from build123d import *

# Parameters (mm, degrees)
SKETCH_1_W             = 580
SKETCH_1_H             = 285
EXTRUDE_1_DEPTH        = 10
HOLE_WIZARD_M5_1_D     = 4.2
HOLE_WIZARD_M5_2_D     = 4.2
HOLE_WIZARD_M5_3_D     = 4.2
SKETCH_11_W            = 330
SKETCH_11_H            = 80
CUT_EXTRUDE_1_DEPTH    = 2
HOLE_WIZARD_M5_4_D     = 4.2
HOLE_WIZARD_M5_4_DEPTH = 2
HOLE_WIZARD_M5_4_TIP   = 1.2618073


with BuildPart() as part:
    # 草图1 → 凸台-拉伸1 (new body)
    with BuildSketch(Plane.XY):
        Rectangle(SKETCH_1_W, SKETCH_1_H)
    extrude(amount=EXTRUDE_1_DEPTH)

    # M5 螺纹孔1 (through all)
    with Locations(Plane(origin=(290, 0, 0), x_dir=(0, 0, -1), z_dir=(1, 0, 0))):
        with Locations((-5, 125), (-5, 75), (-5, 25), (-5, -25), (-5, -75), (-5, -125)):
            Hole(HOLE_WIZARD_M5_1_D / 2)

    # M5 螺纹孔2 (through all)
    with Locations(Plane(origin=(0, 142.5, 0), x_dir=(1, 0, 0), z_dir=(0, 1, 0))):
        with Locations((0, -5), (50, -5)):
            Hole(HOLE_WIZARD_M5_2_D / 2)

    # M5 螺纹孔3 (through all)
    with Locations(Plane.XY.offset(10)):
        with Locations((-160, -132.5), (-80, -132.5), (80, -132.5), (160, -132.5)):
            Hole(HOLE_WIZARD_M5_3_D / 2)

    # 草图11 → 切除-拉伸1 (cut)
    with BuildSketch(Plane(origin=(0, 0, 0), x_dir=(-1, 0, 0), z_dir=(0, 0, -1))):
        with Locations((0, 87.5)):
            Rectangle(SKETCH_11_W, SKETCH_11_H)
    extrude(amount=-CUT_EXTRUDE_1_DEPTH, mode=Mode.SUBTRACT)

    # M5 螺纹孔4
    with Locations(Plane(origin=(0, 0, 2), x_dir=(-1, 0, 0), z_dir=(0, 0, -1))):
        with Locations((-155, 119.5), (-155, 55.5), (155, 55.5), (155, 119.5)):
            Hole(HOLE_WIZARD_M5_4_D / 2, depth=HOLE_WIZARD_M5_4_DEPTH)
            with Locations((0, 0, -(HOLE_WIZARD_M5_4_DEPTH + HOLE_WIZARD_M5_4_TIP / 2))):  # 118° drill point
                Cone(0, HOLE_WIZARD_M5_4_D / 2, HOLE_WIZARD_M5_4_TIP, mode=Mode.SUBTRACT)


solid = part.part
Design review of the part built by this model. Coordinates are the model's own, in mm. Coordinates: 2 decimals unless noted, no trailing zeros. Write each loop counter-clockwise with the first axis right and the second up, starting at its lowest first coordinate (ties: lowest second). Pieces come first, ordered by that corner, then holes. Notation, with made-up numbers: (25, 74) -> (61, 74) arc R18 cw to (61, 98) -> close; hole circle Ø4 at (4.5, 15.25). An arc over 180 degrees is marked (long way). Write each question's results on one line, items separated by ' | '. Start each with the question number.
(1) Take a section at A-A on x = 213.5. Write out the cut boundary in (y, z).
(2) For line 1 along Y through (x, z) = (-155, 2.65); line 2 along X through (y, z) = (78, 0.5); line 3 along Z through (x, y) = (18, -25), list the stretches that pass through material, from the lowest coordinate up. Write a range as from..to.
(3) The part is to be moulded in two halves that separate along Y. For faces 1 (the face through (-4, 142.5, 5)), 2 (the face through (2, 88, 2)), 3 (the face through (-4, 2, 0)), say which applies: pulls with the +Y half, pulls with the -Y half, needs draft (parallel to the pull), parting line crosses it, or undercut.
(4) Take a section at B-B on x = -11. Write out the cut boundary in (y, z), and give its area (3 significant figures).
(5) Clearance check with a flat-ended pin moving along its axis: P1, Ø4, axis at x = 0, z = 5, coming from the +Y side. State where the tip first meets the part, or that it passes through.
Results found:
1) outline: (-142.5, 0) -> (142.5, 0) -> (142.5, 10) -> (-142.5, 10) -> close; hole circle Ø4.2 at (-125, 5); hole circle Ø4.2 at (-75, 5); hole circle Ø4.2 at (-25, 5); hole circle Ø4.2 at (25, 5); hole circle Ø4.2 at (75, 5); hole circle Ø4.2 at (125, 5)
2) line 1: y = -142.5..53.4, 57.6..117.4, 121.6..142.5 | line 2: x = -290..-165, 165..290 | line 3: z = 0..2.9, 7.1..10
3) face 1: pulls with the +Y half | face 2: undercut | face 3: needs draft
4) outline: (-142.5, 0) -> (47.5, 0) -> (47.5, 2) -> (127.5, 2) -> (127.5, 0) -> (142.5, 0) -> (142.5, 10) -> (-142.5, 10) -> close; hole circle Ø4.2 at (-125, 5); hole circle Ø4.2 at (-75, 5); hole circle Ø4.2 at (-25, 5); hole circle Ø4.2 at (25, 5); hole circle Ø4.2 at (75, 5); hole circle Ø4.2 at (125, 5) | area: 2,610 mm2
5) P1: passes through
